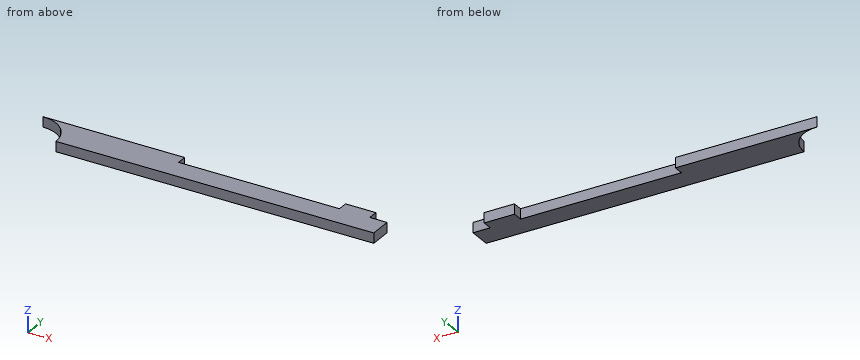
```python
from build123d import *

# Parameters (mm, degrees)
SKETCH1_W           = 15
SKETCH1_H           = 5
BOSS_EXTRUDE1_DEPTH = 2.5


with BuildPart() as part:
    # Sketch1 → Boss-Extrude1 (new, symmetric)
    with BuildSketch(Plane.XY):
        with BuildLine():
            Line((70, 10.875), (30, 10.875))
            Line((30, 10.875), (11.565033506, 10.875))
            ThreePointArc((11.565033506, 10.875), (14.75822706, 5.848962219), (15.875, 0))
            Line((15.875, 0), (173, 0))
            Line((173, 0), (173, 10.875))
            Line((173, 10.875), (164.5, 10.875))
            Line((164.5, 10.875), (149.5, 10.875))
            Line((149.5, 10.875), (70, 10.875))
        make_face()
        with Locations((157, 13.375)):
            Rectangle(SKETCH1_W, SKETCH1_H)
        with BuildLine():
            Line((11.565033506, 10.875), (30, 10.875))
            Line((30, 10.875), (70, 10.875))
            Line((70, 10.875), (70, 15.875))
            Line((70, 15.875), (0, 15.875))
            ThreePointArc((0, 15.875), (6.299801584, 14.571483281), (11.565033506, 10.875))
        make_face()
    extrude(amount=BOSS_EXTRUDE1_DEPTH, both=True)


solid = part.part
```
Work out the finished part from the listing and answer in its coordinate system (mm). Coordinates: 2 decimals unless noted, no trailing zeros. Loops run counter-clockwise (first coordinate to the right, second up) from the corner with the lowest first, then second, coordinate; pieces in that order, holes last.
1) Section C-C (x = 78) is taken. Give the vertices of the cut face in (y, z) (3 decimals).
Results:
outline: (0, -2.5) - (10.875, -2.5) - (10.875, 2.5) - (0, 2.5) - close
2) Flat-ended cylindrical pins translate along their axes: pin 1 (1.5 mm diameter, centred on y = 12.5, z = 0, fed in from -X); pin 2 (2.5 mm diameter, centred on x = 169.5, z = -0.5, fed in from +Y) (3 decimals). Find the tip coordinate at first contact, or state that the pin passes through.
Results:
pin 1: stops at x = 8.74
pin 2: stops at y = 10.875
3) Consider probe 1 along Y at (x, z) = (137.5, -0.1) (3 decimals); probe 2 along X at (y, z) = (0.75, 0.3); probe 3 along X at (y, z) = (14, 1.75). Determine where each line is inside the solid, lowest interval first.
Results:
probe 1: y = 0 to 10.875
probe 2: x = 15.86 to 173
probe 3: x = 7.48 to 70, 149.5 to 164.5
4) Section B-B (z = -0.2) is taken. Give the vertices of the cut face in (x, y) (3 decimals).
Results:
outline: (0, 15.875) arc R15.875 cw to (15.875, 0) - (173, 0) - (173, 10.875) - (164.5, 10.875) - (164.5, 15.875) - (149.5, 15.875) - (149.5, 10.875) - (70, 10.875) - (70, 15.875) - close
5) Section D-D (y = 2.5) is taken. Give the vertices of the cut face in (x, z), plus the area to 3 significant figures.
Results:
outline: (15.68, -2.5) - (173, -2.5) - (173, 2.5) - (15.68, 2.5) - close
area: 787 mm2
6) Section A-A (y = 14) is taken. Give the vertices of the cut face in (x, z), plus the area to 3 significant figures.
Results:
outline: (7.48, -2.5) - (70, -2.5) - (70, 2.5) - (7.48, 2.5) - close; (149.5, -2.5) - (164.5, -2.5) - (164.5, 2.5) - (149.5, 2.5) - close
area: 388 mm2
